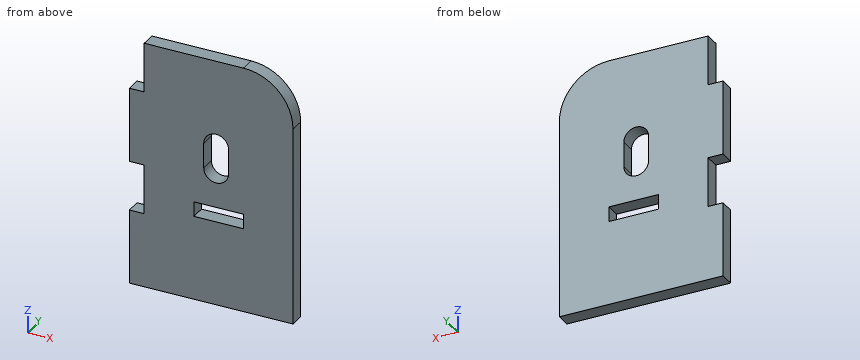
from build123d import *

# Parameters (mm, degrees)
SKETCH1_W           = 10
SKETCH1_H           = 3
BOSS_EXTRUDE1_DEPTH = 3
CUT_EXTRUDE1_DEPTH  = 60.983331018
FILLET1_R           = 10


with BuildPart() as part:
    # Sketch1 → Boss-Extrude1 (new body)
    with BuildSketch(Plane(origin=(0, 0, 0), x_dir=(1, 0, 0), z_dir=(0, 1, 0))):
        Polygon((-33, 0), (-33, -15), (-30, -15), (-30, -25), (-33, -25), (-33, -40), (-30, -40), (-30, -50), (0, -50), (0, 0), align=None)
        with Locations((-15, -18.5)):
            Rectangle(SKETCH1_W, SKETCH1_H, mode=Mode.SUBTRACT)
    extrude(amount=BOSS_EXTRUDE1_DEPTH)

    # Sketch2 → Cut-Extrude1 (cut, through all)
    with BuildSketch(Plane(origin=(0, 3, 0), x_dir=(1, 0, 0), z_dir=(0, 1, 0))):
        with BuildLine():
            Line((-18, -32.5), (-18, -27.5))
            ThreePointArc((-18, -27.5), (-15.5, -25), (-13, -27.5))
            Line((-13, -27.5), (-13, -32.5))
            ThreePointArc((-13, -32.5), (-15.5, -35), (-18, -32.5))
        make_face()
    extrude(amount=-CUT_EXTRUDE1_DEPTH, mode=Mode.SUBTRACT)

    # Fillet1
    fillet1_edges = [part.edges().sort_by_distance(p)[0] for p in [
        (0, 1.5, 50),
    ]]
    fillet(fillet1_edges, radius=FILLET1_R)


solid = part.part
Geometry check sheet. Reference: the model listing, model coordinates, mm. Round coordinates to 2 decimals unless told otherwise and drop trailing zeros. Order: outer loops, then holes, each group sorted by start corner. A loop starts at its lowest first (then second) coordinate and runs counter-clockwise, first axis right, second up. Notation, with made-up numbers: M 81.5,77.5 L 119.5,77.5 A25 cw 119.5,102.5 Z; hole C 23.25,7.5 d8. An arc over 180 degrees is marked long. Answer in a Markdown table with one row per item.
(1) Scan lines: probe 1 along Z at (x, y) = (-12.5, 2.95); probe 2 along Z at (x, y) = (-15, 2.15); probe 3 along X at (y, z) = (0.3, 28). Record each from-to range of solid material in increasing order. Write a range as from..to.
Responses:
| item | result |
|---|---|
| probe 1 | z = 0..17, 20..50 |
| probe 2 | z = 0..17, 20..25.05, 34.95..50 |
| probe 3 | x = -33..-18, -13..0 |
(2) Sectioned sample at B-B, the plane x = -11.5. Record the cut outline in (y, z).
Responses:
| item | result |
|---|---|
| outline | M 0,0 L 3,0 L 3,17 L 0,17 Z; M 0,20 L 3,20 L 3,50 L 0,50 Z |
(3) Go/stop test with flat-tipped pins: P1, Ø1.5, axis at y = 1, z = 18.5, coming from the -X side; P2, Ø0.9, axis at x = -31, y = 2, coming from the +Z side. Record where each tip stops, or that it passes through.
Responses:
| item | result |
|---|---|
| P1 | stops at x = -30 |
| P2 | stops at z = 40 |
(4) Sectioned sample at D-D, the plane x = -4. Record the cut outline in (y, z), and give its area (3 significant figures).
Responses:
| item | result |
|---|---|
| outline | M 0,0 L 3,0 L 3,48 L 0,48 Z |
| area | 144 mm² |
(5) Sectioned sample at C-C, the plane y = 0.95. Record the cut outline in (x, z).
Responses:
| item | result |
|---|---|
| outline | M -33,0 L 0,0 L 0,40 A10 ccw -10,50 L -30,50 L -30,40 L -33,40 L -33,25 L -30,25 L -30,15 L -33,15 Z; hole M -20,17 L -10,17 L -10,20 L -20,20 Z; hole M -18,27.5 A2.5 ccw -13,27.5 L -13,32.5 A2.5 ccw -18,32.5 Z |
(6) Sectioned sample at A-A, the plane x = -15.5. Record the cut outline in (y, z).
Responses:
| item | result |
|---|---|
| outline | M 0,0 L 3,0 L 3,17 L 0,17 Z; M 0,20 L 3,20 L 3,25 L 0,25 Z; M 0,35 L 3,35 L 3,50 L 0,50 Z |
